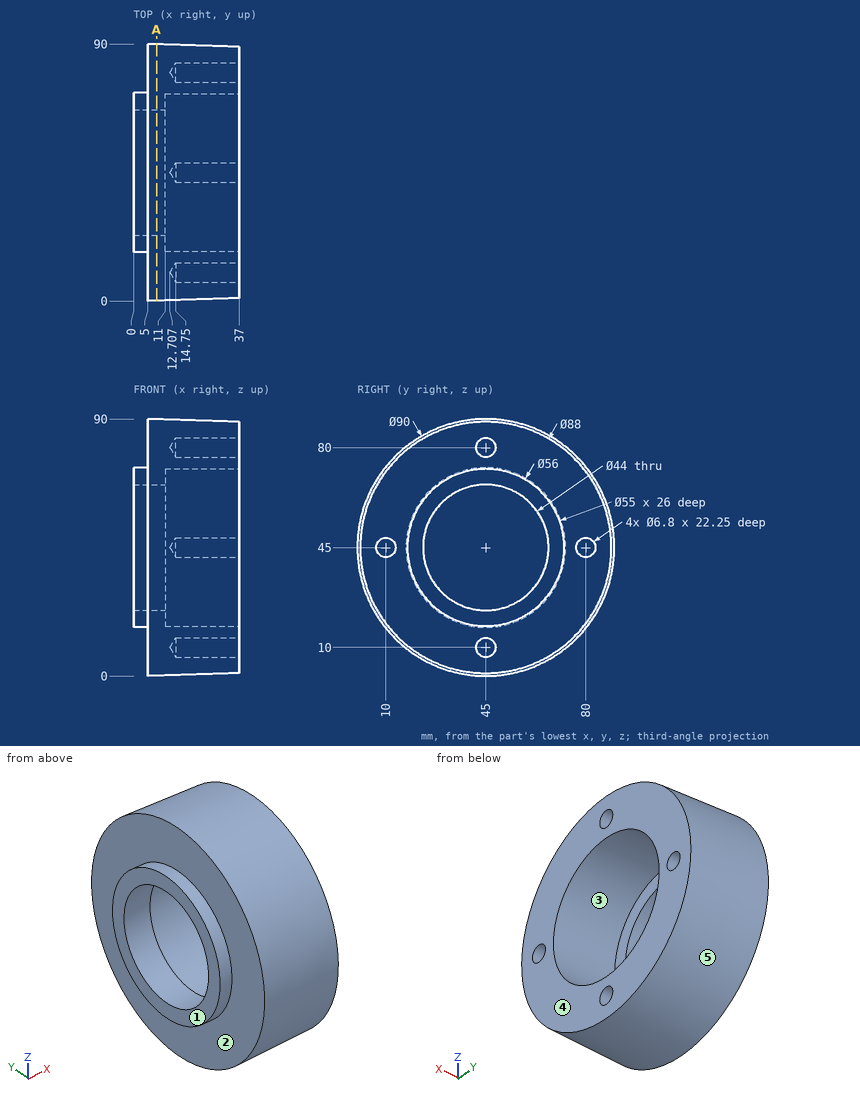
The figure shows three views and two pictorial views of one solid part (mm, origin at its lowest corner). Answer the questions. A direction names the side the tool comes from. Give positions to 0.01 mm unless a question says otherwise; leave off trailing zeros. Loops run counter-clockwise (first coordinate to the right, second up) from the corner with the lowest first, then second, coordinate; pieces in that order, holes last. Notation, with made-up numbers: (74, 72) - (129, 72) arc R26 ccw to (129, 90) - close; hole circle Ø5 at (21, 21). An arc over 180 degrees is marked (long way). Answer in a Markdown table with one row per item.
(1) A tool of negligible diameter and unlimited length cuts with its end or side. For the marked faces 1 and 2, from which of +Z, -Z, +X, -X, +Y, -Y can it reach the whole face along a straight path? Write none if from no direction.
Results list:
| item | result |
|---|---|
| face 1 | +Z, -Z, -X, +Y, -Y |
| face 2 | -X |
(2) Consider L1, parallel to Y at x = 2.5, z = 45; L2, parallel to Y at x = 31.5, z = 45; L3, parallel to Y at x = 32.5, z = 48. Determine where each line is inside the solid, lowest interval first. Write a range as [from, to].
Results list:
| item | result |
|---|---|
| L1 | y = [17, 23], [67, 73] |
| L2 | y = [0.83, 6.6], [13.4, 17.5], [72.5, 76.6], [83.4, 89.17] |
| L3 | y = [0.96, 8.4], [11.6, 17.66], [72.34, 78.4], [81.6, 89.04] |
(3) Section A-A (x = 8) is taken. Give the vertices of the cut face in (y, z), and give its area (3 significant figures).
Results list:
| item | result |
|---|---|
| outline | circle Ø89.81 at (45, 45); hole circle Ø44 at (45, 45) |
| area | 4,810 mm² |
(4) Flat-ended cylindrical pins translate along their axes: pin 1 Ø1.5 at (x, y) = (9.5, 60) entering from +Z; pin 2 Ø4 at (x, z) = (21, 63) entering from +Y; pin 3 Ø10 at (x, y) = (16, 43) entering from -Z. Find the tip coordinate at first contact, or state that the pin passes through.
Results list:
| item | result |
|---|---|
| pin 1 | stops at z = 87.54 |
| pin 2 | stops at y = 86.53 |
| pin 3 | stops at z = 0.2 |
(5) For a pull along Y with two mould halves and no side action, classify the marked faces 3, 4 and 5 as pulls with the +Y half, pulls with the -Y half, needs draft (parallel to the pull), parting line crosses it, or undercut.
Results list:
| item | result |
|---|---|
| face 3 | undercut |
| face 4 | needs draft |
| face 5 | parting line crosses it |
